Design review of the part built by this model. Coordinates are the model's own, in mm. A direction names the side the tool comes from. Coordinates: 2 decimals unless noted, no trailing zeros. Write each loop counter-clockwise with the first axis right and the second up, starting at its lowest first coordinate (ties: lowest second). Pieces come first, ordered by that corner, then holes. Notation, with made-up numbers: (33.5, -34) - (91.5, -34) arc R24 cw to (91.5, -18) - close; hole circle Ø3 at (-22.5, 9.25). An arc over 180 degrees is marked (long way). One line per item, written item: value.
from build123d import *

# Parameters (mm, degrees)
BOSS_EXTRUDE1_DEPTH             = 440
BOSS_EXTRUDE2_DEPTH             = 440
BOSS_EXTRUDE3_DEPTH             = 4
SKETCH4_W                       = 500
SKETCH4_H                       = 4
CUT_EXTRUDE1_DEPTH              = 2
CUT_EXTRUDE3_DEPTH              = 1
CUT_EXTRUDE3_DEPTH_BACK         = 1
CUT_EXTRUDE6_DEPTH              = 54
BOSS_EXTRUDE6_DEPTH             = 40
BOSS_EXTRUDE5_DEPTH             = 40
CUT_EXTRUDE9_DEPTH              = 4
SKETCH14_W                      = 100
SKETCH14_H                      = 100
CUT_EXTRUDE10_DEPTH             = 931.23222907
FILLET1_R                       = 7
FILLET2_R                       = 8
CUT_EXTRUDE11_DEPTH             = 2
SKETCH17_W                      = 40
SKETCH17_H                      = 10
CUT_EXTRUDE12_DEPTH             = 10
SKETCH18_W                      = 44
SKETCH18_H                      = 14
SKETCH18_W_2                    = 40
SKETCH18_H_2                    = 10
BOSS_EXTRUDE7_DEPTH             = 436
CUT_EXTRUDE13_REACH             = 944.28
SKETCH19_W                      = 40
SKETCH19_H                      = 10
CUT_EXTRUDE13_DIRECTION_2_DEPTH = 2
SKETCH20_W                      = 44
SKETCH20_H                      = 14
SKETCH20_W_2                    = 40
SKETCH20_H_2                    = 10
BOSS_EXTRUDE8_DEPTH             = 16
SKETCH21_R                      = 10
CUT_EXTRUDE14_DEPTH             = 25
SKETCH25_R                      = 12
SKETCH25_R_2                    = 10
BOSS_EXTRUDE10_DEPTH            = 17
SKETCH22_R                      = 10
CUT_EXTRUDE15_DEPTH             = 4
SKETCH23_R                      = 12
SKETCH23_R_2                    = 10
BOSS_EXTRUDE9_DEPTH             = 436


with BuildPart() as part:
    # Sketch1 → Boss-Extrude1 (new body)
    with BuildSketch(Plane(origin=(0, 0, 0), x_dir=(1, 0, 0), z_dir=(0, 1, 0))):
        Polygon((0, 300), (-600, 300), (-600, -300), (0, -300), (0, -304), (-604, -304), (-604, 304), (0, 304), align=None)
    extrude(amount=BOSS_EXTRUDE1_DEPTH)



with BuildPart() as body_2:
    # Sketch2 → Boss-Extrude2 (new body)
    with BuildSketch(Plane(origin=(0, 0, 0), x_dir=(1, 0, 0), z_dir=(0, 1, 0))):
        Polygon((0, 250), (-550, 250), (-550, -250), (0, -250), (0, -254), (-554, -254), (-554, 254), (0, 254), align=None)
    extrude(amount=BOSS_EXTRUDE2_DEPTH)


with BuildPart() as part_1:
    add(part.part)

    add(body_2.part)  # Boss-Extrude3 merges body 2
    # Sketch3 → Boss-Extrude3 (add)
    with BuildSketch(Plane(origin=(0, 0, 0), x_dir=(1, 0, 0), z_dir=(0, 1, 0))):
        Polygon((0, -254), (0, -300), (-600, -300), (-600, 300), (0, 300), (0, 254), (-554, 254), (-554, -254), align=None)
    extrude(amount=BOSS_EXTRUDE3_DEPTH)

    # Sketch4 → Cut-Extrude1 (cut)
    with BuildSketch(Plane(origin=(-550, 0, 0), x_dir=(0, 0, -1), z_dir=(1, 0, 0))):
        with Locations((0, 218)):
            Rectangle(SKETCH4_W, SKETCH4_H)
    extrude(amount=-CUT_EXTRUDE1_DEPTH, mode=Mode.SUBTRACT)

    # Sketch7 → Cut-Extrude3 (cut, two sides)
    with BuildSketch(Plane(origin=(0, 64, 0), x_dir=(1, 0, 0), z_dir=(0, 1, 0))) as cut_extrude3_sk:
        Polygon((-550, 250), (0, 250), (0, 252), (-552, 252), (-552, -252), (0, -252), (0, -250), (-550, -250), align=None)
    extrude(amount=CUT_EXTRUDE3_DEPTH, mode=Mode.SUBTRACT)
    extrude(cut_extrude3_sk.sketch, amount=-CUT_EXTRUDE3_DEPTH_BACK, mode=Mode.SUBTRACT)

    # Sketch10 → Cut-Extrude6 (cut)
    with BuildSketch(Plane.XY.offset(304)):
        Polygon((0, 390), (-550, 390), (-550, 220), (-552, 220), (-552, 216), (-550, 216), (-550, 75), (0, 75), align=None)
    extrude(amount=-CUT_EXTRUDE6_DEPTH, mode=Mode.SUBTRACT)

    # Sketch11 → Boss-Extrude6 (add)
    with BuildSketch(Plane(origin=(0, 0, 0), x_dir=(0, 0, -1), z_dir=(1, 0, 0))):
        Polygon((-295, 4), (-295, 19), (-300, 19), (-300, 21), (-293, 21), (-293, 4), align=None)
    extrude(amount=-BOSS_EXTRUDE6_DEPTH)

    # Sketch12 → Boss-Extrude5 (add)
    with BuildSketch(Plane(origin=(0, 0, 0), x_dir=(0, 0, -1), z_dir=(1, 0, 0))):
        Polygon((295, 4), (293, 4), (293, 21), (300, 21), (300, 19), (295, 19), align=None)
    extrude(amount=-BOSS_EXTRUDE5_DEPTH)

    # Sketch13 → Cut-Extrude9 (cut)
    with BuildSketch(Plane.XY.offset(304)):
        with BuildLine():
            Line((0, 400), (0, 430))
            Line((0, 430), (-350, 430))
            ThreePointArc((-350, 430), (-365, 415), (-350, 400))
            Line((-350, 400), (0, 400))
        make_face()
    extrude(amount=-CUT_EXTRUDE9_DEPTH, mode=Mode.SUBTRACT)

    # Sketch14 → Cut-Extrude10 (cut, through all)
    with BuildSketch(Plane.XY.offset(-250)):
        with Locations((-300, 340)):
            Rectangle(SKETCH14_W, SKETCH14_H)
    extrude(amount=-CUT_EXTRUDE10_DEPTH, mode=Mode.SUBTRACT)

    # Fillet1
    fillet1_edges = [part_1.edges().sort_by_distance(p)[0] for p in [
        (-350, 290, -302),
        (-350, 290, -252),
        (-350, 390, -302),
        (-350, 390, -252),
        (-250, 390, -302),
        (-250, 390, -252),
        (-250, 290, -302),
        (-250, 290, -252),
    ]]
    fillet(fillet1_edges, radius=FILLET1_R)

    # Fillet2
    fillet2_edges = [part_1.edges().sort_by_distance(p)[0] for p in [
        (-604, 220, -304),
    ]]
    fillet(fillet2_edges, radius=FILLET2_R)

    # Sketch15 → Cut-Extrude11 (cut)
    with BuildSketch(Plane.XZ):
        Polygon((-600, 300), (-600, 288), (-598, 288), (-598, 298), (-588, 298), (-588, 300), align=None)
    cut_extrude11 = extrude(amount=-CUT_EXTRUDE11_DEPTH, mode=Mode.SUBTRACT)

    # Mirror1: Cut-Extrude11 across plane
    add(cut_extrude11.mirror(Plane.XY), mode=Mode.SUBTRACT)

    # Sketch17 → Cut-Extrude12 (cut)
    with BuildSketch(Plane(origin=(0, 4, 0), x_dir=(1, 0, 0), z_dir=(0, 1, 0))):
        with Locations((-520, 277)):
            Rectangle(SKETCH17_W, SKETCH17_H)
    extrude(amount=-CUT_EXTRUDE12_DEPTH, mode=Mode.SUBTRACT)

    # Sketch18 → Boss-Extrude7 (add)
    with BuildSketch(Plane(origin=(0, 4, 0), x_dir=(1, 0, 0), z_dir=(0, 1, 0))):
        with Locations((-520, 277)):
            Rectangle(SKETCH18_W, SKETCH18_H)
        with Locations((-520, 277)):
            Rectangle(SKETCH18_W_2, SKETCH18_H_2, mode=Mode.SUBTRACT)
    extrude(amount=BOSS_EXTRUDE7_DEPTH)

    # Cut-Extrude13: up to this face of the body (flat: up to its plane)
    cut_extrude13_end = Plane(part_1.part.faces().sort_by_distance((-273.743044457, 248.059881287, -250))[0])
    # Sketch19 → Cut-Extrude13 (cut, up to the picked face)
    with BuildSketch(Plane.XY.offset(-270), mode=Mode.PRIVATE) as cut_extrude13_sk1:
        with Locations((-520, 24)):
            Rectangle(SKETCH19_W, SKETCH19_H)
    cut_extrude13_tool1 = split(extrude(cut_extrude13_sk1.sketch, amount=CUT_EXTRUDE13_REACH, mode=Mode.PRIVATE), bisect_by=cut_extrude13_end, keep=Keep.BOTH, mode=Mode.PRIVATE)
    add(cut_extrude13_tool1.solids().sort_by(Axis((-520, 24, -270), (0, 0, 1)))[0], mode=Mode.SUBTRACT)

    # Sketch19 → Cut-Extrude13 direction 2 (cut)
    with BuildSketch(Plane.XY.offset(-270)):
        with Locations((-520, 24)):
            Rectangle(SKETCH19_W, SKETCH19_H)
    extrude(amount=-CUT_EXTRUDE13_DIRECTION_2_DEPTH, mode=Mode.SUBTRACT)

    # Sketch20 → Boss-Extrude8 (add)
    with BuildSketch(Plane.XY.offset(-270)):
        with Locations((-520, 24)):
            Rectangle(SKETCH20_W, SKETCH20_H)
        with Locations((-520, 24)):
            Rectangle(SKETCH20_W_2, SKETCH20_H_2, mode=Mode.SUBTRACT)
    extrude(amount=BOSS_EXTRUDE8_DEPTH)

    # Sketch21 → Cut-Extrude14 (cut)
    with BuildSketch(Plane.XY.offset(-250)):
        with Locations((-100, 85)):
            Circle(SKETCH21_R)
    extrude(amount=-CUT_EXTRUDE14_DEPTH, mode=Mode.SUBTRACT)

    # Sketch25 → Boss-Extrude10 (add)
    with BuildSketch(Plane(origin=(0, 0, -254), x_dir=(-1, 0, 0), z_dir=(0, 0, -1))):
        with Locations(Location((100, 85, 0), (0, 0, 180))):
            Circle(SKETCH25_R)
        with Locations(Location((100, 85, 0), (0, 0, 180))):
            Circle(SKETCH25_R_2, mode=Mode.SUBTRACT)
    extrude(amount=BOSS_EXTRUDE10_DEPTH)

    # Sketch22 → Cut-Extrude15 (cut)
    with BuildSketch(Plane(origin=(0, 4, 0), x_dir=(1, 0, 0), z_dir=(0, 1, 0))):
        with Locations(Location((-100, 275, 0), (0, 0, 270))):
            Circle(SKETCH22_R)
    extrude(amount=-CUT_EXTRUDE15_DEPTH, mode=Mode.SUBTRACT)

    # Sketch23 → Boss-Extrude9 (add)
    with BuildSketch(Plane(origin=(0, 4, 0), x_dir=(1, 0, 0), z_dir=(0, 1, 0))):
        with Locations(Location((-100, 275, 0), (0, 0, 90))):
            Circle(SKETCH23_R)
        with Locations(Location((-100, 275, 0), (0, 0, 270))):
            Circle(SKETCH23_R_2, mode=Mode.SUBTRACT)
    extrude(amount=BOSS_EXTRUDE9_DEPTH)


solid = part_1.part
1. Consider section A-A, the plane y = 415. Write out the cut boundary in (x, z), then the cut area to 3 significant figures.
Answer block:
outline: (-604, -296) arc R8 ccw to (-596, -304) - (0, -304) - (0, -300) - (-600, -300) - (-600, 300) - (-365, 300) - (-365, 304) - (-604, 304) - close; (-554, -254) - (0, -254) - (0, -250) - (-550, -250) - (-550, 250) - (0, 250) - (0, 254) - (-554, 254) - close; (-542, -284) - (-498, -284) - (-498, -270) - (-542, -270) - close; circle Ø24 at (-100, -275); hole (-540, -282) - (-500, -282) - (-500, -272) - (-540, -272) - close; hole circle Ø20 at (-100, -275)
area: 12,500 mm^2
2. Wall thickness on line 1 along Z through (x, y) = (-201.5, 24.5); line 2 along X through (y, z) = (337, -275); line 3 along X through (y, z) = (85, -255.5): over which ranges is each line inside the solid? List them lowest first.
Answer block:
line 1: z = -304 to -300, -254 to -250, 250 to 254, 300 to 304
line 2: x = -604 to -600, -542 to -540, -500 to -498, -112 to -110, -90 to -88
line 3: x = -604 to -600, -112 to -110, -90 to -88
3. Consider section C-C, the plane z = -42. Write out the cut boundary in (x, y).
Answer block:
outline: (-604, 0) - (-550, 0) - (-550, 63) - (-552, 63) - (-552, 65) - (-550, 65) - (-550, 216) - (-552, 216) - (-552, 220) - (-550, 220) - (-550, 440) - (-554, 440) - (-554, 4) - (-600, 4) - (-600, 440) - (-604, 440) - close
4. For faces 3 (the face through (-520, 219, -284)), 4 (the face through (-20, 11, 295)), 5 (the face through (-365, 415, 302)), 6 (the face through (-550, 31, -3)), list the 3-axis set-ups (+Z, -Z, +X, -X, +Y, -Y) from which the entire face can be reached by the end or side of a thin tool; tool diameter is ignored.
Answer block:
face 3: +Y
face 4: +X
face 5: +Z, +X
face 6: +X, +Y, -Y
5. Insertion check: pin 1 Ø24 at (y, z) = (122.5, -265) entering from +X; pin 2 Ø3 at (y, z) = (62.5, -234) entering from +X; pin 3 Ø12 at (x, y) = (-191, 114.5) entering from +Z. Each pin has a flat end and moves straight along its axis. Give the tip position at first contact, or say it passes through.
Answer block:
pin 1: stops at x = 0
pin 2: stops at x = -550
pin 3: stops at z = -250
6. Consider section B-B, the plane x = -472. Give the number of separate pieces and of enclosed holes in the cut face, then the cut area to 3 significant figures.
Answer block:
separate pieces: 4
enclosed holes: 0
area: 4,880 mm^2
7. Mouldability with a two-part tool opening along Y and no side actions: class faces 1 (the face through (-520, 17, -262)), 2 (the face through (-520, 217, -282)) as released by +Y, released by -Y, zero draft, split by the parting line, or undercut.
Answer block:
face 1: undercut
face 2: zero draft
